The model under review builds one solid part; all positions refer to its coordinate system, in mm. A direction names the side the tool comes from. Round coordinates to 2 decimals unless told otherwise and drop trailing zeros. Loops run counter-clockwise (first coordinate to the right, second up) from the corner with the lowest first, then second, coordinate; pieces in that order, holes last. Notation, with made-up numbers: (16, 60) -> (59, 60) arc R15 cw to (59, 82) -> close; hole circle Ø6 at (45.25, -37.5). An arc over 180 degrees is marked (long way). Return JSON: item names as keys, results as strings. Group by question number.
```python
from build123d import *

# Parameters (mm, degrees)
SALIENTE_EXTRUIR1_DEPTH = 40
CROQUIS2_W              = 9.479166667
CROQUIS2_H              = 25
CROQUIS2_W_2            = 25
CROQUIS2_H_2            = 9.479166667
SALIENTE_EXTRUIR2_DEPTH = 80
CROQUIS3_R              = 20
SALIENTE_EXTRUIR3_DEPTH = 80
CROQUIS4_R              = 15
CORTAR_EXTRUIR1_DEPTH   = 80
CROQUIS8_W              = 4
CROQUIS8_H              = 3
SALIENTE_EXTRUIR4_DEPTH = 19
CROQUIS9_R              = 15
CORTAR_EXTRUIR3_DEPTH   = 363.429876335


with BuildPart() as part:
    # Croquis1 → Saliente-Extruir1 (new, symmetric)
    with BuildSketch(Plane.XY):
        with BuildLine():
            ThreePointArc((-224.955926351, -4.453223482), (-159.292265632, -158.90555091), (-5, -224.944437584))
            ThreePointArc((-5, -224.944437584), (72.506901641, -212.997063863), (141.205472177, -175.174240764))
            ThreePointArc((141.205472177, -175.174240764), (145.300285764, -171.79297703), (149.31416044, -168.316016742))
            ThreePointArc((149.31416044, -168.316016742), (204.039526473, -94.83075259), (224.929799791, -5.620068165))
            ThreePointArc((224.929799791, -5.620068165), (224.982449263, -2.810253291), (225, 0))
            ThreePointArc((225, 0), (224.982449263, 2.810253291), (224.929799791, 5.620068165))
            ThreePointArc((224.929799791, 5.620068165), (204.170039134, 94.549432151), (149.777577039, 167.903774277))
            ThreePointArc((149.777577039, 167.903774277), (145.536932266, 171.592544554), (141.205472177, 175.174240764))
            ThreePointArc((141.205472177, 175.174240764), (77.513474556, 211.226563818), (5.620068165, 224.929799791))
            ThreePointArc((5.620068165, 224.929799791), (0.310120458, 224.999786278), (-5, 224.944437584))
            ThreePointArc((-5, 224.944437584), (-77.513474556, 211.226563818), (-141.687825127, 174.784324843))
            ThreePointArc((-141.687825127, 174.784324843), (-202.138767057, 98.817603962), (-224.955926351, 4.453223482))
            ThreePointArc((-224.955926351, 4.453223482), (-225, 0), (-224.955926351, -4.453223482))
        make_face()
        with BuildLine():
            ThreePointArc((-5, -214.941852602), (-74.312911497, -201.748831929), (-135.622478375, -166.827885437))
            Line((-135.622478375, -166.827885437), (-5.334401385, -14.019420882))
            ThreePointArc((-5.334401385, -14.019420882), (-5.16756497, -14.081770921), (-5, -14.142135624))
            Line((-5, -14.142135624), (-5, -214.941852602))
        make_face(mode=Mode.SUBTRACT)
        with BuildLine():
            Line((-12.960736698, -7.551112781), (-142.45440376, -161.033359431))
            ThreePointArc((-142.45440376, -161.033359431), (-195.095815172, -90.347235166), (-214.95333695, -4.479166667))
            Line((-214.95333695, -4.479166667), (-14.142135624, -5))
            ThreePointArc((-14.142135624, -5), (-13.611335942, -6.303295477), (-12.960736698, -7.551112781))
        make_face(mode=Mode.SUBTRACT)
        with BuildLine():
            ThreePointArc((135.622478375, -166.827885437), (74.068431242, -201.838716537), (4.479166667, -214.95333695))
            Line((4.479166667, -214.95333695), (5, -14.142135624))
            ThreePointArc((5, -14.142135624), (5.16756497, -14.081770921), (5.334401385, -14.019420882))
            Line((5.334401385, -14.019420882), (135.622478375, -166.827885437))
        make_face(mode=Mode.SUBTRACT)
        with BuildLine():
            Line((142.844180294, -160.687710035), (12.960736698, -7.551112781))
            ThreePointArc((12.960736698, -7.551112781), (13.611335942, -6.303295477), (14.142135624, -5))
            Line((14.142135624, -5), (214.95333695, -4.479166667))
            ThreePointArc((214.95333695, -4.479166667), (195.205130803, -90.110803505), (142.844180294, -160.687710035))
        make_face(mode=Mode.SUBTRACT)
        with BuildLine():
            ThreePointArc((-214.95333695, 4.479166667), (-195.095815172, 90.347235166), (-142.45440376, 161.033359431))
            Line((-142.45440376, 161.033359431), (-12.960736698, 7.551112781))
            ThreePointArc((-12.960736698, 7.551112781), (-13.611335942, 6.303295477), (-14.142135624, 5))
            Line((-14.142135624, 5), (-214.95333695, 4.479166667))
        make_face(mode=Mode.SUBTRACT)
        with BuildLine():
            Line((-5.334401385, 14.019420882), (-135.21784498, 167.156018135))
            ThreePointArc((-135.21784498, 167.156018135), (-74.068431242, 201.838716537), (-5, 214.941852602))
            Line((-5, 214.941852602), (-5, 14.142135624))
            ThreePointArc((-5, 14.142135624), (-5.16756497, 14.081770921), (-5.334401385, 14.019420882))
        make_face(mode=Mode.SUBTRACT)
        with BuildLine():
            Line((214.95333695, 4.479166667), (14.142135624, 5))
            ThreePointArc((14.142135624, 5), (13.611335942, 6.303295477), (12.960736698, 7.551112781))
            Line((12.960736698, 7.551112781), (142.45440376, 161.033359431))
            ThreePointArc((142.45440376, 161.033359431), (195.095815172, 90.347235166), (214.95333695, 4.479166667))
        make_face(mode=Mode.SUBTRACT)
        with BuildLine():
            ThreePointArc((5.334401385, 14.019420882), (5.16756497, 14.081770921), (5, 14.142135624))
            Line((5, 14.142135624), (4.479166667, 214.95333695))
            ThreePointArc((4.479166667, 214.95333695), (74.068431242, 201.838716537), (135.622478375, 166.827885437))
            Line((135.622478375, 166.827885437), (5.334401385, 14.019420882))
        make_face(mode=Mode.SUBTRACT)
    extrude(amount=SALIENTE_EXTRUIR1_DEPTH, both=True)

    # Croquis2 → Saliente-Extruir2 (add)
    with BuildSketch(Plane.XY.offset(40)):
        Polygon((90.224919325, 206.117597339), (99.792005134, 229.214585652), (91.034397066, 232.842105688), (81.467311257, 209.745117375), align=None)
        with Locations((-0.260416666, 237.455411284)):
            Rectangle(CROQUIS2_W, CROQUIS2_H)
        Polygon((162.234745908, 155.900247659), (179.912415437, 173.577917189), (173.209632407, 180.280700219), (155.531962878, 162.603030689), align=None)
        Polygon((209.545803087, 81.948498513), (232.6427914, 91.515584322), (229.015271364, 100.273192391), (205.918283051, 90.706106582), align=None)
        with Locations((237.455411284, 0.260416666)):
            Rectangle(CROQUIS2_W_2, CROQUIS2_H_2)
        Polygon((206.117597339, -90.224919325), (229.214585652, -99.792005134), (232.842105688, -91.034397066), (209.745117375, -81.467311257), align=None)
        Polygon((155.90024766, -162.234745908), (173.577917189, -179.912415437), (180.280700219, -173.209632407), (162.603030689, -155.531962878), align=None)
        Polygon((81.948498513, -209.545803087), (91.515584322, -232.6427914), (100.273192391, -229.015271364), (90.706106582, -205.918283051), align=None)
        with Locations((0.260416666, -237.455411284)):
            Rectangle(CROQUIS2_W, CROQUIS2_H)
        Polygon((-90.224919325, -206.117597339), (-99.792005134, -229.214585652), (-91.034397066, -232.842105688), (-81.467311257, -209.745117375), align=None)
        Polygon((-162.234745908, -155.900247659), (-179.912415437, -173.577917189), (-173.209632407, -180.280700219), (-155.531962878, -162.603030689), align=None)
        Polygon((-209.545803087, -81.948498513), (-232.6427914, -91.515584322), (-229.015271364, -100.273192391), (-205.918283051, -90.706106582), align=None)
        with Locations((-237.455411284, -0.260416666)):
            Rectangle(CROQUIS2_W_2, CROQUIS2_H_2)
        Polygon((-206.117597339, 90.224919325), (-229.214585652, 99.792005134), (-232.842105688, 91.034397066), (-209.745117375, 81.467311257), align=None)
        Polygon((-155.900247659, 162.234745908), (-173.577917189, 179.912415437), (-180.280700219, 173.209632407), (-162.603030689, 155.531962878), align=None)
        Polygon((-81.948498513, 209.545803087), (-91.515584322, 232.6427914), (-100.273192391, 229.015271364), (-90.706106582, 205.918283051), align=None)
    extrude(amount=-SALIENTE_EXTRUIR2_DEPTH)

    # Croquis3 → Saliente-Extruir3 (add)
    with BuildSketch(Plane(origin=(0, 0, -40), x_dir=(-1, 0, 0), z_dir=(0, 0, -1))):
        Circle(CROQUIS3_R)
    extrude(amount=-SALIENTE_EXTRUIR3_DEPTH)

    # Croquis4 → Cortar-Extruir1 (cut)
    with BuildSketch(Plane(origin=(0, 0, -40), x_dir=(-1, 0, 0), z_dir=(0, 0, -1))):
        Circle(CROQUIS4_R)
    extrude(amount=-CORTAR_EXTRUIR1_DEPTH, mode=Mode.SUBTRACT)

    # Croquis8 → Saliente-Extruir4 (add)
    with BuildSketch(Plane(origin=(0, 0, -40), x_dir=(-1, 0, 0), z_dir=(0, 0, -1))):
        with Locations((0, 15)):
            Rectangle(CROQUIS8_W, CROQUIS8_H)
    extrude(amount=SALIENTE_EXTRUIR4_DEPTH)

    # Croquis9 → Cortar-Extruir3 (cut, through all)
    with BuildSketch(Plane(origin=(0, 0, -40), x_dir=(-1, 0, 0), z_dir=(0, 0, -1))):
        with Locations(Location((0, 0, 0), (0, 0, 82.337744339))):
            Circle(CROQUIS9_R)
    extrude(amount=CORTAR_EXTRUIR3_DEPTH, mode=Mode.SUBTRACT)


solid = part.part
```
1. Tool access review of faces 1 (the face through (-94.94, -217.5, 0.56)), 2 (the face through (-5, 237, 1)), 3 (the face through (-73.1, -93.5, -0.6)): name each direction out of +Z, -Z, +X, -X, +Y, -Y from which nothing blocks a thin tool from reaching the whole face with its end or side.
2. Draft analysis for pull direction X (two halves, no side actions). For faces 4 (the face through (164.495, 171.566, 0.56)), 5 (the face through (-221.46, 86.32, 0.56)), 6 (the face through (170.95, 164.615, 0.56)), state which applies: pulls with the +X half, pulls with the -X half, needs draft (parallel to the pull), parting line crosses it, or undercut.
3. We need section D-D, the plane x = -27. Write out the cut boundary in (y, z), then the cut area to 3 significant figures.
4. For P1, Ø1.5, axis at x = -66.5, z = -37.5, coming from the +Y side; P2, Ø7.5, axis at y = 241.5, z = -11.5, coming from the -X side; P3, Ø1.3, axis at y = 15.5, z = -46.5, coming from the -X side, all flat-tipped, find the tip position at first contact; note any pin that passes through.
5. We need section B-B, the plane x = 75. Write out the cut boundary in (y, z).
6. Wall thickness on line 1 (X direction, y = 0, z = 1); line 2 (X direction, y = 82.5, z = 23): over which ranges is each line inside the solid? List them lowest first.
7. We need section C-C, the plane z = 24. Give the number of separate pieces and of enclosed holes in the cut face, then the cut area to 3 significant figures.
8. We need section A-A, the plane y = -195. Write out the cut boundary in (x, z), then the cut area to 3 significant figures.
Check sheet entries:
{
 "1": {"face 1": "+Z, -Z, -X", "face 2": "+Z, -Z, +Y", "face 3": "+Z, -Z"},
 "2": {"face 4": "undercut", "face 5": "pulls with the -X half", "face 6": "pulls with the +X half"},
 "3": {"outline": "(-223.37, -40) -> (-213.3, -40) -> (-213.3, 40) -> (-223.37, 40) -> close; (-39.43, -40) -> (-24.19, -40) -> (-24.19, 40) -> (-39.43, 40) -> close; (-4.97, -40) -> (4.97, -40) -> (4.97, 40) -> (-4.97, 40) -> close; (24.19, -40) -> (39.56, -40) -> (39.56, 40) -> (24.19, 40) -> close; (213.3, -40) -> (223.37, -40) -> (223.37, 40) -> (213.3, 40) -> close", "area": "4,860 mm²"},
 "4": {"P1": "stops at y = 215.18", "P2": "stops at x = -5", "P3": "stops at x = -2"},
 "5": {"outline": "(-212.13, -40) -> (-201.49, -40) -> (-201.49, 40) -> (-212.13, 40) -> close; (-95.73, -40) -> (-80.7, -40) -> (-80.7, 40) -> (-95.73, 40) -> close; (-4.84, -40) -> (4.84, -40) -> (4.84, 40) -> (-4.84, 40) -> close; (81.08, -40) -> (95.73, -40) -> (95.73, 40) -> (81.08, 40) -> close; (201.49, -40) -> (212.13, -40) -> (212.13, 40) -> (201.49, 40) -> close"},
 "6": {"line 1": "x = -249.96 to -15, 15 to 249.96", "line 2": "x = -212.24 to -198.54, -76.2 to -63.42, -5 to 4.82, 63.72 to 76.2, 198.54 to 210.88"},
 "7": {"separate pieces": "1", "enclosed holes": "9", "area": "33,100 mm²"},
 "8": {"outline": "(-112.25, -40) -> (-90.55, -40) -> (-90.55, 40) -> (-112.25, 40) -> close; (-5, -40) -> (4.53, -40) -> (4.53, 40) -> (-5, 40) -> close; (90.55, -40) -> (112.25, -40) -> (112.25, 40) -> (90.55, 40) -> close", "area": "4,230 mm²"}
}
